Part print with two shaded views. Sizes in mm from the minimum x, y, z corner. A direction names the side the tool comes from. Coordinates: 2 decimals unless noted, no trailing zeros. Write each loop counter-clockwise with the first axis right and the second up, starting at its lowest first coordinate (ties: lowest second). Pieces come first, ordered by that corner, then holes.
Q1. Pull direction X, two halves, no side cores. Call the marked faces 1, 2 and 3: released by +X, released by -X, zero draft, split by the parting line, or undercut.
Q2. Band-saw the part on B-B, the plane x = 33.5. Write the cut outline in (y, z), plus the area to 3 significant figures.
Q3. Drill centre lines: probe 1 along Z at (x, y) = (2.5, 0.9); probe 2 along X at (y, z) = (2.5, 9.5); probe 3 along X at (y, z) = (1.25, 6.25). Where is each one in solid material? Low to high.
Q4. Pin check, flat tips, straight feed: P1, Ø5, axis at x = 14, z = 6.5, coming from the -Y side; P2, Ø4, axis at x = 34, z = 5, coming from the +Y side; P3, Ø4, axis at y = 10, z = 2, coming from the -X side. Stop position of each tip, or through.
Q5. Band-saw the part on D-D, the plane z = 3.5. Write the cut outline in (x, y).
Q6. Band-saw the part on A-A, the plane z = 5. Write the cut outline in (x, y), plus the area to 3 significant figures.
Q7. Which spindle directions (+Z, -Z, +X, -X, +Y, -Y) get a long thin tool onto all of the face, cutting with end or side? Do the marked faces 4, 5, 6 and 7. Say none if no direction does.
Q8. Band-saw the part on C-C, the plane y = 6. Write the cut outline in (x, z), plus the area to 3 significant figures.
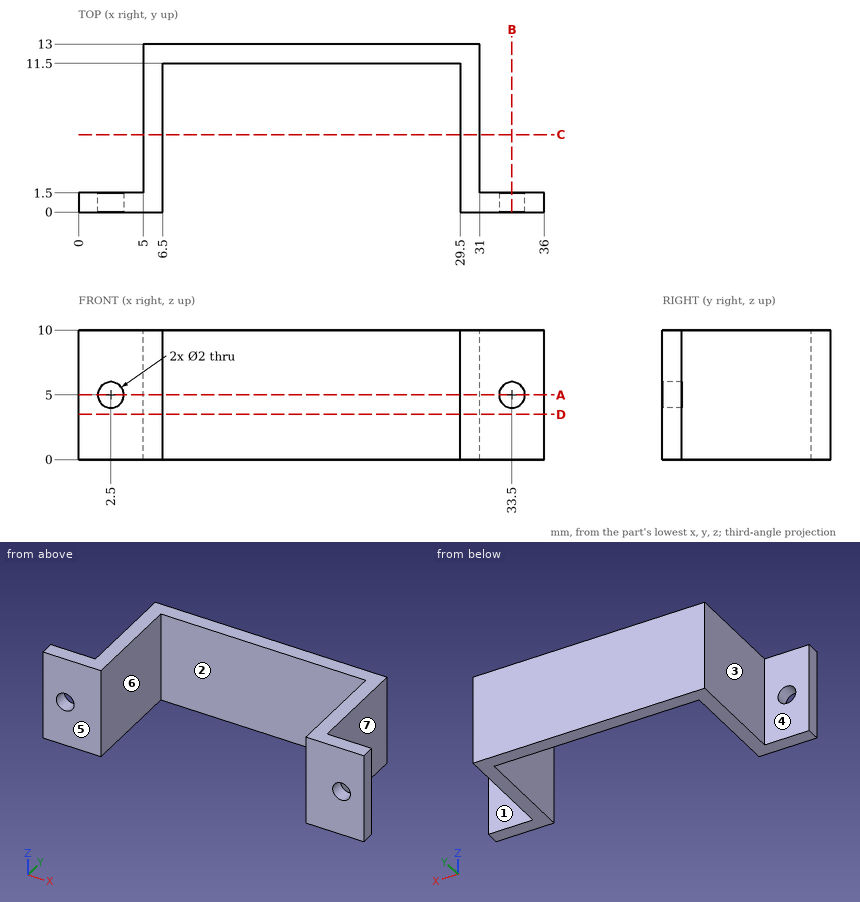
Answer sheet:
1. face 1: zero draft
1. face 2: undercut
1. face 3: released by -X
2. outline: (0, 0) - (1.5, 0) - (1.5, 4) - (0, 4) - close; (0, 6) - (1.5, 6) - (1.5, 10) - (0, 10) - close
2. area: 12.0 mm2
3. probe 1: z = 0 to 4, 6 to 10
3. probe 2: x = 5 to 6.5, 29.5 to 31
3. probe 3: x = 0 to 6.5, 29.5 to 36
4. P1: stops at y = 11.5
4. P2: stops at y = 1.5
4. P3: stops at x = 5
5. outline: (0, 0) - (6.5, 0) - (6.5, 11.5) - (29.5, 11.5) - (29.5, 0) - (36, 0) - (36, 1.5) - (31, 1.5) - (31, 13) - (5, 13) - (5, 1.5) - (0, 1.5) - close
6. outline: (0, 0) - (1.5, 0) - (1.5, 1.5) - (0, 1.5) - close; (3.5, 0) - (6.5, 0) - (6.5, 11.5) - (29.5, 11.5) - (29.5, 0) - (32.5, 0) - (32.5, 1.5) - (31, 1.5) - (31, 13) - (5, 13) - (5, 1.5) - (3.5, 1.5) - close; (34.5, 0) - (36, 0) - (36, 1.5) - (34.5, 1.5) - close
6. area: 82.5 mm2
7. face 4: +Z, -Z, -X, +Y
7. face 5: +Z, -Z, +X, -X, -Y
7. face 6: +Z, -Z, -Y
7. face 7: +Z, -Z, +X, +Y
8. outline: (5, 0) - (6.5, 0) - (6.5, 10) - (5, 10) - close; (29.5, 0) - (31, 0) - (31, 10) - (29.5, 10) - close
8. area: 30.0 mm2
